Check sheet for the drawn part. Datum: minimum x, y, z corner. Units: mm. A direction names the side the tool comes from. Give positions to 0.01 mm unless a question says otherwise; leave off trailing zeros. Order: outer loops, then holes, each group sorted by start corner. A loop starts at its lowest first (then second) coordinate and runs counter-clockwise, first axis right, second up.
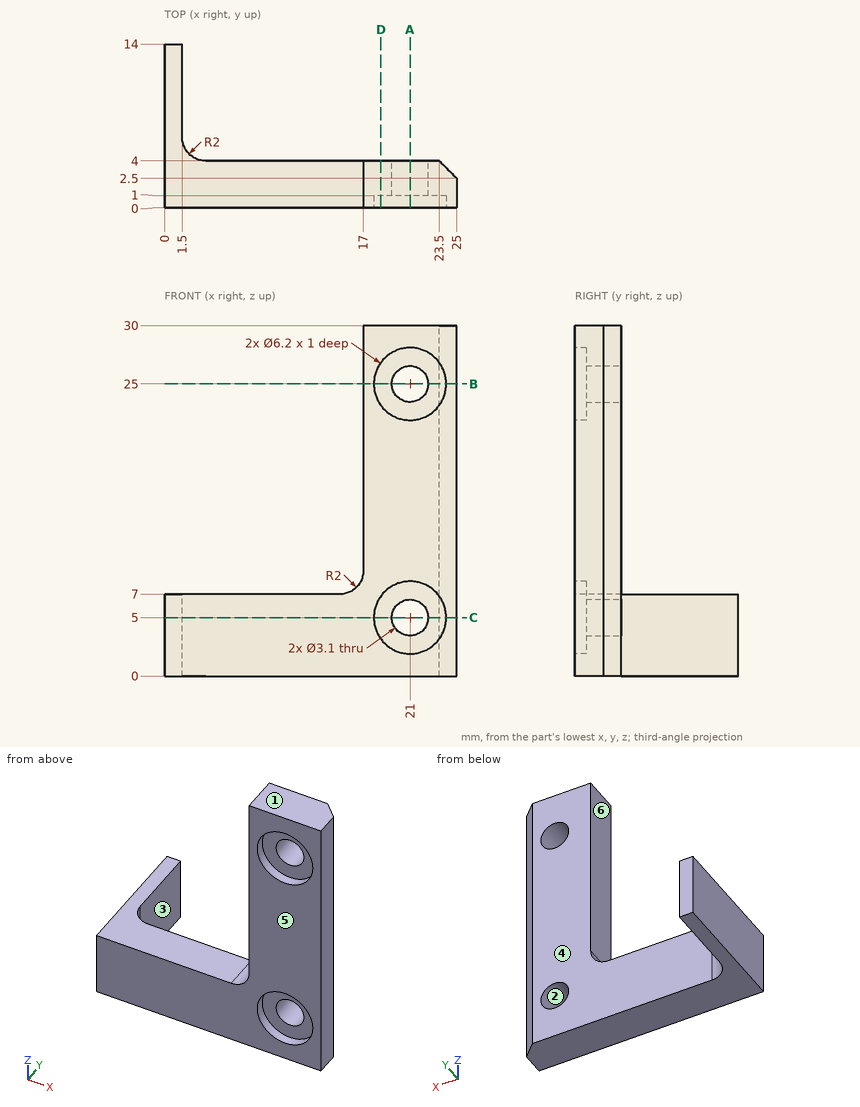
Q1. Sectioned sample at C-C, the plane z = 5. Record the cut outline in (x, y), plus the area to 3 significant figures.
Q2. Tool access check on the marked faces 4, 5 and 6. Record the directions out of +Z, -Z, +X, -X, +Y, -Y that give a thin tool (end or side, any length) a straight path to the whole face; none if there is none.
Q3. Go/stop test with flat-tipped pins: P1, Ø3.5, axis at x = 21, z = 25, coming from the +Y side; P2, Ø3, axis at y = 9.5, z = 9, coming from the -X side; P3, Ø5, axis at x = 20.5, z = 25, coming from the -Y side; P4, Ø2, axis at y = 9.5, z = 5, coming from the +X side. Record where each tip stops, or that it passes through.
Q4. Material ranges on line 1 (Z direction, x = 21, y = 0.8); line 2 (Z direction, x = 21, y = 1.65); line 3 (Y direction, x = 23.25, z = 26), recorded low to high.
Q5. Sectioned sample at A-A, the plane x = 21. Record the cut outline in (y, z), plus the area to 3 significant figures.
Q6. Sectioned sample at D-D, the plane x = 18.5. Record the cut outline in (y, z), plus the area to 3 significant figures.
Q7. Draft check along X on the marked faces 1, 2 and 3. Enter one of: pulls with the +X half, pulls with the -X half, needs draft (parallel to the pull), parting line crosses it, or undercut.
Q8. Sectioned sample at B-B, the plane z = 25. Record the cut outline in (x, y), plus the area to 3 significant figures.
Filled in:
1. outline: (0, 0) - (17.9, 0) - (17.9, 1) - (19.45, 1) - (19.45, 4) - (3.5, 4) arc R2 cw to (1.5, 6) - (1.5, 14) - (0, 14) - close; (22.55, 1) - (24.1, 1) - (24.1, 0) - (25, 0) - (25, 2.5) - (23.5, 4) - (22.55, 4) - close
1. area: 99.2 mm2
2. face 4: +Z, -Z, +X, +Y
2. face 5: +Z, -Z, +X, -X, -Y
2. face 6: +Z, -X, +Y, -Y
3. P1: stops at y = 4
3. P2: passes through
3. P3: stops at y = 1
3. P4: stops at x = 1.5
4. line 1: z = 0 to 1.9, 8.1 to 21.9, 28.1 to 30
4. line 2: z = 0 to 3.45, 6.55 to 23.45, 26.55 to 30
4. line 3: y = 1 to 4
5. outline: (0, 0) - (4, 0) - (4, 3.45) - (1, 3.45) - (1, 1.9) - (0, 1.9) - close; (0, 8.1) - (1, 8.1) - (1, 6.55) - (4, 6.55) - (4, 23.45) - (1, 23.45) - (1, 21.9) - (0, 21.9) - close; (0, 28.1) - (1, 28.1) - (1, 26.55) - (4, 26.55) - (4, 30) - (0, 30) - close
5. area: 89.0 mm2
6. outline: (0, 0) - (4, 0) - (4, 30) - (0, 30) - (0, 26.83) - (1, 26.83) - (1, 23.17) - (0, 23.17) - (0, 6.83) - (1, 6.83) - (1, 3.17) - (0, 3.17) - close
6. area: 113 mm2
7. face 1: needs draft
7. face 2: undercut
7. face 3: pulls with the +X half
8. outline: (17, 0) - (17.9, 0) - (17.9, 1) - (19.45, 1) - (19.45, 4) - (17, 4) - close; (22.55, 1) - (24.1, 1) - (24.1, 0) - (25, 0) - (25, 2.5) - (23.5, 4) - (22.55, 4) - close
8. area: 15.4 mm2
